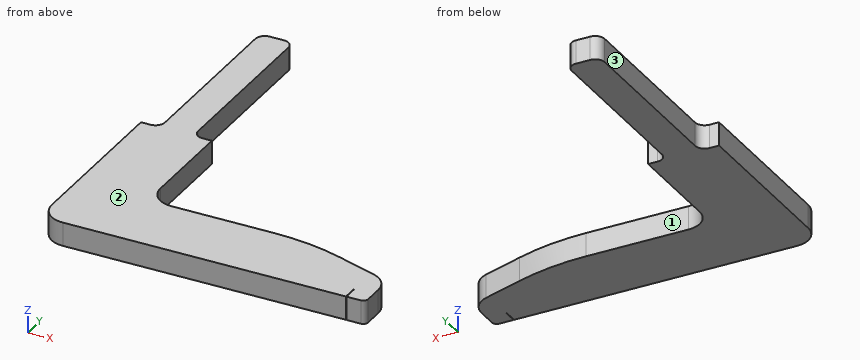
from build123d import *

# Parameters (mm, degrees)
BOSS_EXTRUDE1_DEPTH = 5
SKETCH2_W           = 0.1
SKETCH2_H           = 5
CUT_EXTRUDE2_DEPTH  = 3
FILLET1_R           = 2


with BuildPart() as part:
    # Sketch1 → Boss-Extrude1 (new body)
    with BuildSketch(Plane.XY):
        with BuildLine():
            Line((0, -1), (0, -35.5))
            ThreePointArc((0, -35.5), (1.464466094, -39.035533906), (5, -40.5))
            Line((5, -40.5), (68, -40.5))
            ThreePointArc((68, -40.5), (68.707106781, -40.207106781), (69, -39.5))
            Line((69, -39.5), (69, -35.429996046))
            ThreePointArc((69, -35.429996046), (68.042547906, -32.487580979), (65.53687743, -30.672054499))
            Line((65.53687743, -30.672054499), (57.01873992, -27.920584529))
            ThreePointArc((57.01873992, -27.920584529), (49.429079532, -26.108853154), (41.649965621, -25.5))
            Line((41.649965621, -25.5), (20, -25.5))
            ThreePointArc((20, -25.5), (16.464466094, -24.035533906), (15, -20.5))
            Line((15, -20.5), (15, -1))
            Line((15, -1), (15, 0))
            Line((15, 0), (14, 0))
            Line((14, 0), (11, 0))
            Line((11, 0), (11, 40))
            Line((11, 40), (4, 40))
            Line((4, 40), (4, 0))
            Line((4, 0), (1, 0))
            Line((1, 0), (0, 0))
            Line((0, 0), (0, -1))
        make_face()
    extrude(amount=BOSS_EXTRUDE1_DEPTH)

    # Sketch2 → Cut-Extrude2 (cut)
    with BuildSketch(Plane.XZ.offset(40.5)):
        with Locations((64.9, 2.5)):
            Rectangle(SKETCH2_W, SKETCH2_H)
    extrude(amount=-CUT_EXTRUDE2_DEPTH, mode=Mode.SUBTRACT)

    # Fillet1
    fillet1_edges = [part.edges().sort_by_distance(p)[0] for p in [
        (4, 0, 2.5),
        (4, 40, 2.5),
        (11, 40, 2.5),
        (11, 0, 2.5),
    ]]
    fillet(fillet1_edges, radius=FILLET1_R)


solid = part.part
Input: part model. Units: mm. Frame: model coordinates. Face numbers are marked on the shaded views. A direction names the side the tool comes from. Round coordinates to 2 decimals unless told otherwise and drop trailing zeros. Order: outer loops, then holes, each group sorted by start corner. A loop starts at its lowest first (then second) coordinate and runs counter-clockwise, first axis right, second up. Notation, with made-up numbers: (-5.75, -14.75) - (38.25, -14.75) arc R19 ccw to (38.25, 20.25) - close; hole circle Ø6 at (-26, 62.25). An arc over 180 degrees is marked (long way). Answer as a JSON object with one key per item and string values. Group by question number.
(1) Material intervals for probe 1 along X at (y, z) = (34.5, 2.2); probe 2 along Y at (x, z) = (39.5, 1); probe 3 along X at (y, z) = (-2, 4.25), sorted ascending. Write a range as from..to.
(2) Reachability of the marked faces 1, 2 and 3 from +Z, -Z, +X, -X, +Y, -Y: full face, straight path, thin tool, end or side. Return the list, or none.
(3) Cut plane C-C (x = 49). Return loops of the section in (y, z).
(4) Cut plane B-B (x = 29). Return loops of the section in (y, z), then the cut area to 3 significant figures.
(5) Pin query (flat end, axial travel): P1, Ø1, axis at y = 23, z = 2.5, coming from the -X side; P2, Ø2, axis at y = -13, z = 1.5, coming from the +X side; P3, Ø1.5, axis at y = -39, z = 2.5, coming from the -X side. Return the tip coordinate at first contact, or that it passes through.
(6) Cut plane A-A (z = 3.1). Return loops of the section in (x, y), then the cut area to 3 significant figures.
Here are the results:
{
 "1": {"probe 1": "x = 4..11", "probe 2": "y = -40.5..-25.5", "probe 3": "x = 0..15"},
 "2": {"face 1": "+Z, -Z, +X, +Y", "face 2": "+Z, +X, -X, +Y, -Y", "face 3": "+Z, -Z, -X, +Y"},
 "3": {"outline": "(-40.5, 0) - (-26.04, 0) - (-26.04, 5) - (-40.5, 5) - close"},
 "4": {"outline": "(-40.5, 0) - (-25.5, 0) - (-25.5, 5) - (-40.5, 5) - close", "area": "75.0 mm^2"},
 "5": {"P1": "stops at x = 4", "P2": "stops at x = 15", "P3": "stops at x = 0.82"},
 "6": {"outline": "(0, -35.5) arc R5 ccw to (5, -40.5) - (64.85, -40.5) - (64.85, -37.5) - (64.95, -37.5) - (64.95, -40.5) - (68, -40.5) arc R1 ccw to (69, -39.5) - (69, -35.43) arc R5 ccw to (65.54, -30.67) - (57.02, -27.92) arc R50 ccw to (41.65, -25.5) - (20, -25.5) arc R5 cw to (15, -20.5) - (15, 0) - (13, 0) arc R2 cw to (11, 2) - (11, 38) arc R2 ccw to (9, 40) - (6, 40) arc R2 ccw to (4, 38) - (4, 2) arc R2 cw to (2, 0) - (0, 0) - close", "area": "1,630 mm^2"}
}
